```python
from build123d import *

# Parameters (mm, degrees)
BOSS_EXTRUDE1_DEPTH = 4
BOSS_EXTRUDE2_DEPTH = 7.8
SKETCH4_W           = 33.781239108
SKETCH4_H           = 10.810531084
CUT_EXTRUDE1_DEPTH  = 28.88035773
SKETCH6_R           = 1.75
BOSS_EXTRUDE3_DEPTH = 3
FILLET1_R           = 3
CUT_EXTRUDE2_REACH  = 35.305
SKETCH7_R           = 7.75
SKETCH8_R           = 1.75
BOSS_EXTRUDE4_DEPTH = 8.8
BOSS_EXTRUDE5_DEPTH = 2


with BuildPart() as part:
    # Sketch2 → Boss-Extrude1 (new body)
    with BuildSketch(Plane.XY):
        with BuildLine():
            Line((3.481334242, 16.311673717), (-3.481334242, 16.311673717))
            Line((-3.481334242, 16.311673717), (-4.292170887, 16.824998456))
            ThreePointArc((-4.292170887, 16.824998456), (-11.492625639, 13.016253681), (-16.163850494, 6.342967853))
            Line((-16.163850494, 6.342967853), (-16.163850494, -14.391495343))
            Line((-16.163850494, -14.391495343), (-14.353897969, -14.640433541))
            Line((-14.353897969, -14.640433541), (-10.527602773, -17.523753782))
            Line((-10.527602773, -17.523753782), (-10.527602773, -19.404011272))
            Line((-10.527602773, -19.404011272), (-5.007128349, -19.404011272))
            Line((-5.007128349, -19.404011272), (-5.007128349, -17.507596758))
            Line((-5.007128349, -17.507596758), (5, -17.507596758))
            Line((5, -17.507596758), (5, -19.411447251))
            Line((5, -19.411447251), (10.467237067, -19.411447251))
            Line((10.467237067, -19.411447251), (10.467237067, -17.567178369))
            Line((10.467237067, -17.567178369), (14.33922382, -14.64942707))
            Line((14.33922382, -14.64942707), (16.163850494, -14.424396197))
            Line((16.163850494, -14.424396197), (16.163850494, 6.342967853))
            ThreePointArc((16.163850494, 6.342967853), (11.492625639, 13.016253681), (4.292170887, 16.824998456))
            Line((4.292170887, 16.824998456), (3.481334242, 16.311673717))
        make_face()
    extrude(amount=BOSS_EXTRUDE1_DEPTH)

    # Sketch3 → Boss-Extrude2 (add)
    with BuildSketch(Plane.XY.offset(4)):
        with BuildLine():
            Line((4.292170887, 16.824998456), (3.481334242, 16.311673717))
            Line((3.481334242, 16.311673717), (-3.481334242, 16.311673717))
            Line((-3.481334242, 16.311673717), (-4.292170887, 16.824998456))
            ThreePointArc((-4.292170887, 16.824998456), (-11.492625639, 13.016253681), (-16.163850494, 6.342967853))
            Line((-16.163850494, 6.342967853), (-16.163850494, -14.391495343))
            Line((-16.163850494, -14.391495343), (-14.353897969, -14.640433541))
            Line((-14.353897969, -14.640433541), (-10.527602773, -17.523753782))
            Line((-10.527602773, -17.523753782), (-10.527602773, -19.404011272))
            Line((-10.527602773, -19.404011272), (-5.007128349, -19.404011272))
            Line((-5.007128349, -19.404011272), (-5.007128349, -17.507596758))
            Line((-5.007128349, -17.507596758), (5, -17.507596758))
            Line((5, -17.507596758), (5, -19.411447251))
            Line((5, -19.411447251), (10.467237067, -19.411447251))
            Line((10.467237067, -19.411447251), (10.467237067, -17.567178369))
            Line((10.467237067, -17.567178369), (14.33922382, -14.64942707))
            Line((14.33922382, -14.64942707), (16.163850494, -14.424396197))
            Line((16.163850494, -14.424396197), (16.163850494, 6.342967853))
            ThreePointArc((16.163850494, 6.342967853), (11.492625639, 13.016253681), (4.292170887, 16.824998456))
        make_face()
        with BuildLine():
            Line((4.003211271, 14.511673717), (-4.003211271, 14.511673717))
            Line((-4.003211271, 14.511673717), (-4.577751285, 14.875403704))
            ThreePointArc((-4.577751285, 14.875403704), (-10.460467666, 11.524411412), (-14.363850494, 5.992765737))
            Line((-14.363850494, 5.992765737), (-14.363850494, -12.822119288))
            Line((-14.363850494, -12.822119288), (-13.644664568, -12.921035058))
            Line((-13.644664568, -12.921035058), (-8.727602773, -16.626306888))
            Line((-8.727602773, -16.626306888), (-8.727602773, -17.604011272))
            Line((-8.727602773, -17.604011272), (-6.807128349, -17.604011272))
            Line((-6.807128349, -17.604011272), (-6.807128349, -15.707596758))
            Line((-6.807128349, -15.707596758), (6.8, -15.707596758))
            Line((6.8, -15.707596758), (6.8, -17.611447251))
            Line((6.8, -17.611447251), (8.667237067, -17.611447251))
            Line((8.667237067, -17.611447251), (8.667237067, -16.669731475))
            Line((8.667237067, -16.669731475), (13.640731753, -12.921934411))
            Line((13.640731753, -12.921934411), (14.363850494, -12.832752309))
            Line((14.363850494, -12.832752309), (14.363850494, 5.992765737))
            ThreePointArc((14.363850494, 5.992765737), (10.460467666, 11.524411412), (4.577751285, 14.875403704))
            Line((4.577751285, 14.875403704), (4.003211271, 14.511673717))
        make_face(mode=Mode.SUBTRACT)
    extrude(amount=BOSS_EXTRUDE2_DEPTH)

    # Sketch4 → Cut-Extrude1 (cut, through all)
    with BuildSketch(Plane(origin=(0, 0, 0), x_dir=(-1, 0, 0), z_dir=(0, 0, -1))):
        Polygon((-4.606626741, 14.656974178), (-4.606626741, 16.741633553), (-2.485703279, 20.488617531), (2.721605339, 20.671050509), (4.606626741, 16.741633553), (4.606626741, 14.656974178), (4.606626741, 14.311673717), (-4.606626741, 14.311673717), align=None)
        with Locations((0.72676906, -18.06116853)):
            Rectangle(SKETCH4_W, SKETCH4_H)
    extrude(amount=-CUT_EXTRUDE1_DEPTH, mode=Mode.SUBTRACT)

    # Sketch6 → Boss-Extrude3 (add)
    with BuildSketch(Plane.XY.offset(11.8)):
        with BuildLine():
            Line((-16.163850494, -7.542701658), (-16.163850494, 6.342967853))
            Line((-16.163850494, 6.342967853), (-23.929756214, 3.11778647))
            ThreePointArc((-23.929756214, 3.11778647), (-26.262186338, 0.009769983), (-23.948484604, -3.11221353))
            Line((-23.948484604, -3.11221353), (-16.163850494, -7.542701658))
        make_face()
        with Locations((-20, 0)):
            Circle(SKETCH6_R, mode=Mode.SUBTRACT)
        with BuildLine():
            Line((16.163850494, -7.542701658), (16.163850494, 6.342967853))
            Line((16.163850494, 6.342967853), (23.859195057, 3.11778647))
            ThreePointArc((23.859195057, 3.11778647), (26.152039317, 0.046872999), (23.925870502, -3.072712992))
            Line((23.925870502, -3.072712992), (16.163850494, -7.542701658))
        make_face()
        with Locations((20, 0)):
            Circle(SKETCH6_R, mode=Mode.SUBTRACT)
    extrude(amount=-BOSS_EXTRUDE3_DEPTH)

    # Fillet1
    fillet1_edges = [part.edges().sort_by_distance(p)[0] for p in [
        (16.163850494, -7.542701658, 10.3),
        (-16.163850494, -7.542701658, 10.3),
        (16.163850494, 6.342967853, 10.3),
        (-16.163850494, 6.342967853, 10.3),
    ]]
    fillet(fillet1_edges, radius=FILLET1_R)

    # Sketch7 → Cut-Extrude2 (cut, up to next)
    with BuildSketch(Plane(origin=(0, 0, 0), x_dir=(-1, 0, 0), z_dir=(0, 0, -1)), mode=Mode.PRIVATE) as cut_extrude2_sk1:
        Circle(SKETCH7_R)
    cut_extrude2_tool1 = extrude(cut_extrude2_sk1.sketch, amount=-CUT_EXTRUDE2_REACH, mode=Mode.PRIVATE) & part.part
    add(cut_extrude2_tool1.solids().sort_by_distance((0, 0, 0))[0], mode=Mode.SUBTRACT)

    # Sketch8 → Boss-Extrude4 (add)
    with BuildSketch(Plane(origin=(0, 0, 8.8), x_dir=(-1, 0, 0), z_dir=(0, 0, -1))):
        with BuildLine():
            Line((-17.279436212, 5.875416821), (-23.859195057, 3.11778647))
            ThreePointArc((-23.859195057, 3.11778647), (-26.152039317, 0.046872999), (-23.925870502, -3.072712992))
            Line((-23.925870502, -3.072712992), (-17.666718993, -6.677230408))
            ThreePointArc((-17.666718993, -6.677230408), (-16.566602479, -7.775527074), (-16.163850494, -9.276960639))
            Line((-16.163850494, -9.276960639), (-16.163850494, 6.342967853))
            ThreePointArc((-16.163850494, 6.342967853), (-15.951477639, 6.859567413), (-15.722599163, 7.369069108))
            ThreePointArc((-15.722599163, 7.369069108), (-16.362099709, 6.477448451), (-17.279436212, 5.875416821))
        make_face()
        with Locations(Location((-20, 0, 0), (0, 0, 180))):
            Circle(SKETCH8_R, mode=Mode.SUBTRACT)
        with BuildLine():
            Line((17.679948892, -6.679840815), (23.948484604, -3.11221353))
            ThreePointArc((23.948484604, -3.11221353), (26.262186338, 0.009769983), (23.929756214, 3.11778647))
            Line((23.929756214, 3.11778647), (17.285932986, 5.876966887))
            ThreePointArc((17.285932986, 5.876966887), (16.363441184, 6.479081897), (15.720481601, 7.373585437))
            ThreePointArc((15.720481601, 7.373585437), (15.9504922, 6.861858534), (16.163850494, 6.342967853))
            Line((16.163850494, 6.342967853), (16.163850494, -9.287145177))
            ThreePointArc((16.163850494, -9.287145177), (16.570425653, -7.779117459), (17.679948892, -6.679840815))
        make_face()
        with Locations(Location((20, 0, 0), (0, 0, 180))):
            Circle(SKETCH8_R, mode=Mode.SUBTRACT)
    extrude(amount=BOSS_EXTRUDE4_DEPTH)

    # Sketch9 → Boss-Extrude5 (add)
    with BuildSketch(Plane.XZ.offset(12.655902988)):
        Polygon((-16.163850494, 0), (16.163850494, 0), (16.163850494, 11.8), (14.363850494, 11.8), (14.363850494, 4), (-14.363850494, 4), (-14.363850494, 11.8), (-16.163850494, 11.8), align=None)
    extrude(amount=BOSS_EXTRUDE5_DEPTH)


solid = part.part
```
Work out the finished part from the listing and answer in its coordinate system (mm). A direction names the side the tool comes from. Give positions to 0.01 mm unless a question says otherwise; leave off trailing zeros. Loops run counter-clockwise (first coordinate to the right, second up) from the corner with the lowest first, then second, coordinate; pieces in that order, holes last. Notation, with made-up numbers: (25, -19) -> (77, -19) arc R30 ccw to (77, 20) -> close; hole circle Ø4 at (-5, 65.25). An arc over 180 degrees is marked (long way). Use CSV: the item, a comma, the result in double quotes.
1. The part is cut by section D-D (z = 1). Write down the section's boundary in (x, y), then the cut area to 3 significant figures.
Found:
outline,"(-23.95, -3.11) -> (-17.68, -6.68) arc R3 cw to (-16.16, -9.29) -> (-16.16, -14.66) -> (16.16, -14.66) -> (16.16, -9.28) arc R3 cw to (17.67, -6.68) -> (23.93, -3.07) arc R3.25 ccw to (23.86, 3.12) -> (17.28, 5.88) arc R3 cw to (15.72, 7.37) arc R17.36 ccw to (4.61, 16.74) -> (4.61, 14.31) -> (-4.61, 14.31) -> (-4.61, 16.74) arc R17.36 ccw to (-15.72, 7.37) arc R3 cw to (-17.29, 5.88) -> (-23.93, 3.12) arc R3.25 ccw to start; hole circle Ø3.5 at (-20, 0); hole circle Ø15.5 at (0, 0); hole circle Ø3.5 at (20, 0)"
area,"881 mm^2"
2. The part is cut by section B-B (x = 0). Write down the section's boundary in (y, z), then the cut area to 3 significant figures.
Found:
outline,"(-14.66, 0) -> (-7.75, 0) -> (-7.75, 4) -> (-14.66, 4) -> close; (7.75, 0) -> (14.31, 0) -> (14.31, 4) -> (7.75, 4) -> close"
area,"53.9 mm^2"
3. Flat-ended cylindrical pins translate along their axes: pin 1 Ø1 at (y, z) = (-13.5, 8) entering from -X; pin 2 Ø3 at (x, z) = (-2, 2.5) entering from +Y; pin 3 Ø2 at (x, z) = (-18.5, 4.5) entering from +Y. Find the tip coordinate at first contact, or state that the pin passes through.
Found:
pin 1,"x = -16.16"
pin 2,"y = 14.31"
pin 3,"y = 5.79"
4. A tool of negligible diameter and unlimited length cuts with its end or side. For faces 5 (the flat face through (16.164, -12, 6)), 6 (the flat face through (4.607, 16, 6)), 7 (the cylindrical face through (-10.4, 11.58, 7.85)), 8 (the flat face through (-16.164, -12, 6)), 9 (the cylindrical face through (1.009, 7.684, 1.972)), from which of +Z, -Z, +X, -X, +Y, -Y can it reach the whole face along a straight path? Write none if from no direction.
Found:
face 5,"+Z, -Z, +X, -Y"
face 6,"+Z, -Z, +Y"
face 7,"+Z, -Y"
face 8,"+Z, -Z, -X, -Y"
face 9,"+Z, -Z"
5. Straight lines are drawn through the part: line 1 (X direction, y = 0.5, z = 8.5); line 2 (Z direction, x = -7, y = -12.5); line 3 (Y direction, x = 0, z = 2.25). For each, find the intervals that lie inside material, in ascending order.
Found:
line 1,"-26.22 to -21.68, -18.32 to -14.36, 14.36 to 18.32, 21.68 to 26.12"
line 2,"0 to 4"
line 3,"-14.66 to -7.75, 7.75 to 14.31"
6. The part is cut by section C-C (y = -4). Write down the section's boundary in (x, z).
Found:
outline,"(-22.39, 0) -> (-6.64, 0) -> (-6.64, 4) -> (-14.36, 4) -> (-14.36, 11.8) -> (-22.39, 11.8) -> close; (6.64, 0) -> (22.32, 0) -> (22.32, 11.8) -> (14.36, 11.8) -> (14.36, 4) -> (6.64, 4) -> close"
7. The mould has two halves that part along X. Classify faces 1 (the cylindrical face through (-26.26, -0.05, 5.98)), 2 (the cylindrical face through (10.54, 11.45, 7.85)), 3 (the flat face through (-17, 1, 11.8)), 4 (the cylindrical face through (11.27, 13.21, 5.82)): +X half, -X half, draft (parallel to the pull), parting line (faces both ways), or undercut.
Found:
face 1,"-X half"
face 2,"undercut"
face 3,"draft"
face 4,"+X half"
8. The part is cut by section A-A (z = 6.75). Write down the section's boundary in (x, y), then the cut area to 3 significant figures.
Found:
outline,"(-23.95, -3.11) -> (-17.68, -6.68) arc R3 cw to (-16.16, -9.29) -> (-16.16, -14.66) -> (-14.36, -14.66) -> (-14.36, 5.99) arc R15.56 cw to (-4.61, 14.87) -> (-4.61, 16.74) arc R17.36 ccw to (-15.72, 7.37) arc R3 cw to (-17.29, 5.88) -> (-23.93, 3.12) arc R3.25 ccw to start; (4.61, 14.87) arc R15.56 cw to (14.36, 5.99) -> (14.36, -14.66) -> (16.16, -14.66) -> (16.16, -9.28) arc R3 cw to (17.67, -6.68) -> (23.93, -3.07) arc R3.25 ccw to (23.86, 3.12) -> (17.28, 5.88) arc R3 cw to (15.72, 7.37) arc R17.36 ccw to (4.61, 16.74) -> close; hole circle Ø3.5 at (-20, 0); hole circle Ø3.5 at (20, 0)"
area,"287 mm^2"
